Part print with two shaded views. Sizes in mm from the minimum x, y, z corner. A direction names the side the tool comes from. Coordinates: 2 decimals unless noted, no trailing zeros. Write each loop counter-clockwise with the first axis right and the second up, starting at its lowest first coordinate (ties: lowest second). Pieces come first, ordered by that corner, then holes. Notation, with made-up numbers: M 85.25,-19.75 L 134.25,-19.75 A31 cw 134.25,15.25 Z; hole C 23.5,-12.5 d4. An arc over 180 degrees is marked long. Answer in a Markdown table with one row per item. Add a question column.
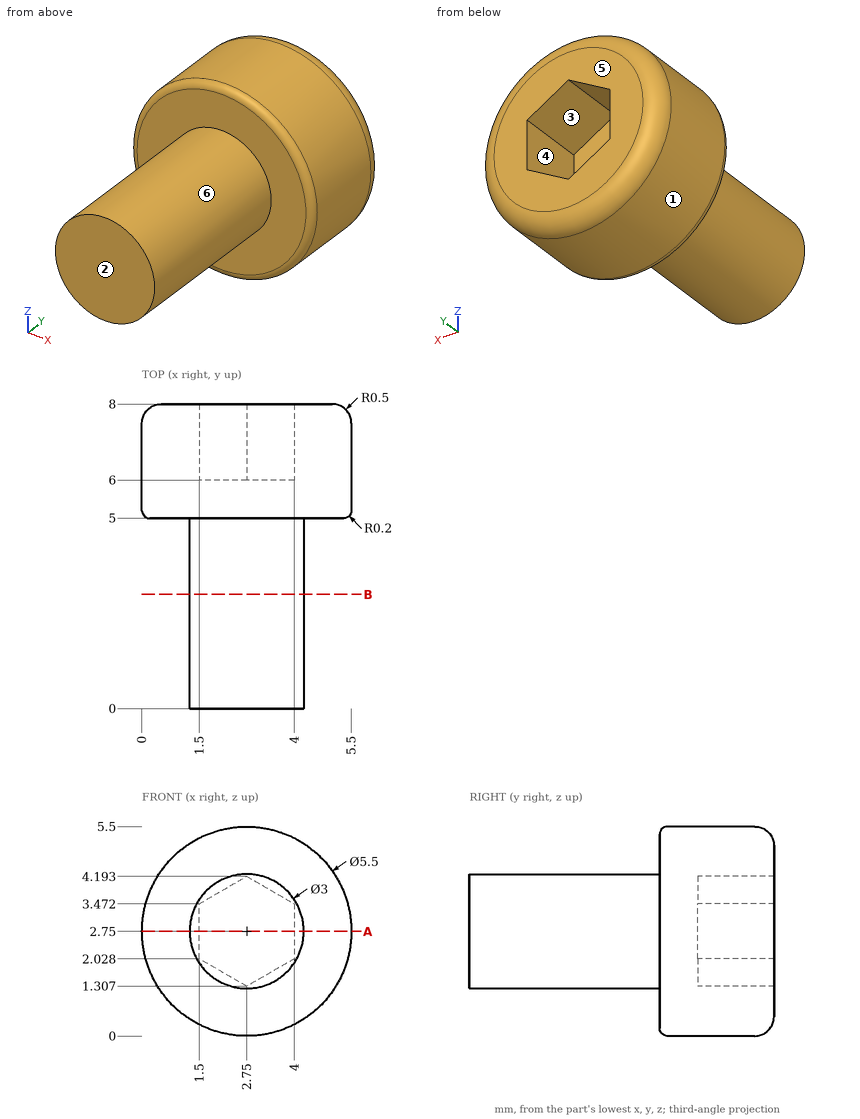
1) Two-plate mould, pull along X, no slides. Class the marked faces 1, 2, 3 and 4: released by +X, released by -X, zero draft, split by the parting line, or undercut.
2) Slice it at A-A (z = 2.75). Give the cut face in (x, y).
3) Which spindle directions (+Z, -Z, +X, -X, +Y, -Y) get a long thin tool onto all of the face, cutting with end or side? Do the marked faces 5 and 6. Say none if no direction does.
4) Slice it at B-B (y = 3). Give the cut face in (x, z).
5) Flat gauge pins, fed straight in: pin 1 Ø2 at (y, z) = (6.5, 1.5) entering from +X; pin 2 Ø2.5 at (x, z) = (2, 4) entering from -Y; pin 3 Ø0.8 at (x, z) = (2.5, 2.5) entering from +Y. Where does each tip first touch, or does it go through?
6) Drill centre lines: probe 1 along X at (y, z) = (1.5, 2.8); probe 2 along Y at (x, z) = (3.4, 4.85); probe 3 along Y at (x, z) = (1.7, 2.1). Where is each one in solid material? Low to high.
Ans:
| question | item | result |
|---|---|---|
| 1 | face 1 | split by the parting line |
| 1 | face 2 | zero draft |
| 1 | face 3 | undercut |
| 1 | face 4 | undercut |
| 2 | outline | M 0,5.2 A0.2 ccw 0.2,5 L 1.25,5 L 1.25,0 L 4.25,0 L 4.25,5 L 5.3,5 A0.2 ccw 5.5,5.2 L 5.5,7.5 A0.5 ccw 5,8 L 4,8 L 4,6 L 1.5,6 L 1.5,8 L 0.5,8 A0.5 ccw 0,7.5 Z |
| 3 | face 5 | +Z, -Z, +X, -X, +Y |
| 3 | face 6 | -Y |
| 4 | outline | C 2.75,2.75 d3 |
| 5 | pin 1 | stops at x = 5.49 |
| 5 | pin 2 | stops at y = 0 |
| 5 | pin 3 | stops at y = 6 |
| 6 | probe 1 | x = 1.25 to 4.25 |
| 6 | probe 2 | y = 5 to 8 |
| 6 | probe 3 | y = 0 to 6 |
